Geometry check sheet. Reference: the model listing, model coordinates, mm. A direction names the side the tool comes from. Coordinates: 2 decimals unless noted, no trailing zeros. Loops run counter-clockwise (first coordinate to the right, second up) from the corner with the lowest first, then second, coordinate; pieces in that order, holes last.
from build123d import *

# Parameters (mm, degrees)
F0_R     = 12.7
F1_DEPTH = 6.35


# Not quite as in the source:
# - a feature of the source that left no trace in its solid (it failed there, or was rolled back) is left out


with BuildPart() as f1:
    # F0 (on Top) → F1 (new body, symmetric)
    with BuildSketch(Plane.XY):
        Polygon((4.1113441396, 43.5372516477), (2.5, 50), (-2.5, 50), (-4.1113441396, 43.5372516477), (-9.5436300128, 42.6768620899), (-13.073208428, 48.3253683007), (-17.8284910095, 46.7802833288), (-17.3638712822, 40.1359116722), (-22.2644071652, 37.6389639237), (-27.3667201287, 41.9203128495), (-31.4118051006, 38.981386588), (-28.9167017225, 32.805789019), (-32.805789019, 28.9167017225), (-38.981386588, 31.4118051006), (-41.9203128495, 27.3667201287), (-37.6389639237, 22.2644071652), (-40.1359116722, 17.3638712822), (-46.7802833288, 17.8284910095), (-48.3253683007, 13.073208428), (-42.6768620899, 9.5436300128), (-43.5372516477, 4.1113441396), (-50, 2.5), (-50, -2.5), (-43.5372516477, -4.1113441396), (-42.6768620899, -9.5436300128), (-48.3253683007, -13.073208428), (-46.7802833288, -17.8284910095), (-40.1359116722, -17.3638712822), (-37.6389639237, -22.2644071652), (-41.9203128495, -27.3667201287), (-38.981386588, -31.4118051006), (-32.805789019, -28.9167017225), (-28.9167017225, -32.805789019), (-31.4118051006, -38.981386588), (-27.3667201287, -41.9203128495), (-22.2644071652, -37.6389639237), (-17.3638712822, -40.1359116722), (-17.8284910095, -46.7802833288), (-13.073208428, -48.3253683007), (-9.5436300128, -42.6768620899), (-4.1113441396, -43.5372516477), (-2.5, -50), (2.5, -50), (4.1113441396, -43.5372516477), (9.5436300128, -42.6768620899), (13.073208428, -48.3253683007), (17.8284910095, -46.7802833288), (17.3638712822, -40.1359116722), (22.2644071652, -37.6389639237), (27.3667201287, -41.9203128495), (31.4118051006, -38.981386588), (28.9167017225, -32.805789019), (32.805789019, -28.9167017225), (38.981386588, -31.4118051006), (41.9203128495, -27.3667201287), (37.6389639237, -22.2644071652), (40.1359116722, -17.3638712822), (46.7802833288, -17.8284910095), (48.3253683007, -13.073208428), (42.6768620899, -9.5436300128), (43.5372516477, -4.1113441396), (50, -2.5), (50, 2.5), (43.5372516477, 4.1113441396), (42.6768620899, 9.5436300128), (48.3253683007, 13.073208428), (46.7802833288, 17.8284910095), (40.1359116722, 17.3638712822), (37.6389639237, 22.2644071652), (41.9203128495, 27.3667201287), (38.981386588, 31.4118051006), (32.805789019, 28.9167017225), (28.9167017225, 32.805789019), (31.4118051006, 38.981386588), (27.3667201287, 41.9203128495), (22.2644071652, 37.6389639237), (17.3638712822, 40.1359116722), (17.8284910095, 46.7802833288), (13.073208428, 48.3253683007), (9.5436300128, 42.6768620899), align=None)
        Circle(F0_R, mode=Mode.SUBTRACT)
    extrude(amount=F1_DEPTH, both=True)


solid = f1.part
(1) Sectioned sample at C-C on x = -34.5. Record the cut outline in (y, z).
Findings:
outline: (-29.6, -6.35) - (29.6, -6.35) - (29.6, 6.35) - (-29.6, 6.35) - close
(2) Sectioned sample at D-D on y = 21. Record the cut outline in (x, z).
Findings:
outline: (-38.28, -6.35) - (38.28, -6.35) - (38.28, 6.35) - (-38.28, 6.35) - close
(3) Gauge pin test, flat ends, axial feed: pin 1 Ø4 at (y, z) = (19.5, -4) entering from +X; pin 2 Ø6 at (y, z) = (-27.5, 1) entering from +X; pin 3 Ø3 at (x, z) = (13, 3) entering from +Y; pin 4 Ø23 at (x, y) = (0, 0) entering from +Z. Record the tip position at first contact, or that the pin passes through.
Findings:
pin 1: stops at x = 46.89
pin 2: stops at x = 41.92
pin 3: stops at y = 48.33
pin 4: passes through
(4) Scan lines: L1, parallel to Y at x = 0, z = 0.5; L2, parallel to Y at x = 29.5, z = 4.75; L3, parallel to X at y = -5, z = 5.5. Record each from-to range of solid material in increasing order.
Findings:
L1: y = -50 to -12.7, 12.7 to 50
L2: y = -40.37 to -34.25, -32.22 to 32.22, 34.25 to 40.37
L3: x = -43.4 to -11.67, 11.67 to 43.4
(5) Access from +Z, -Z, +X, -X, +Y, -Y to the whole of each face (thin tool, end or side, straight path). Record for faces 5 (the flat face through (-35.937, -30.182, 0.089)), 6 (the flat face through (45.541, -11.333, 0.089)), 7 (the flat face through (24.85, 39.81, 0.09)), 8 (the flat face through (17.6, -43.5, 0.1)).
Findings:
face 5: +Z, -Z, -Y
face 6: +Z, -Z, +X
face 7: +Z, -Z, +Y
face 8: +Z, -Z
(6) Sectioned sample at A-A on x = 0. Record the cut outline in (y, z), and give its area (3 significant figures).
Findings:
outline: (-50, -6.35) - (-12.7, -6.35) - (-12.7, 6.35) - (-50, 6.35) - close; (12.7, -6.35) - (50, -6.35) - (50, 6.35) - (12.7, 6.35) - close
area: 947 mm2
(7) Draft check along Y on faces 1 (the flat face through (-3.317, -46.723, 0.089)), 2 (the flat face through (10, -10, 6.35)), 3 (the flat face through (-35.85, 30.147, 0.089)), 4 (the flat face through (-43.5, -17.6, 0.1)). Enter one of: +Y half, -Y half, draft (parallel to the pull), parting line (faces both ways), or undercut.
Findings:
face 1: -Y half
face 2: draft
face 3: +Y half
face 4: undercut
